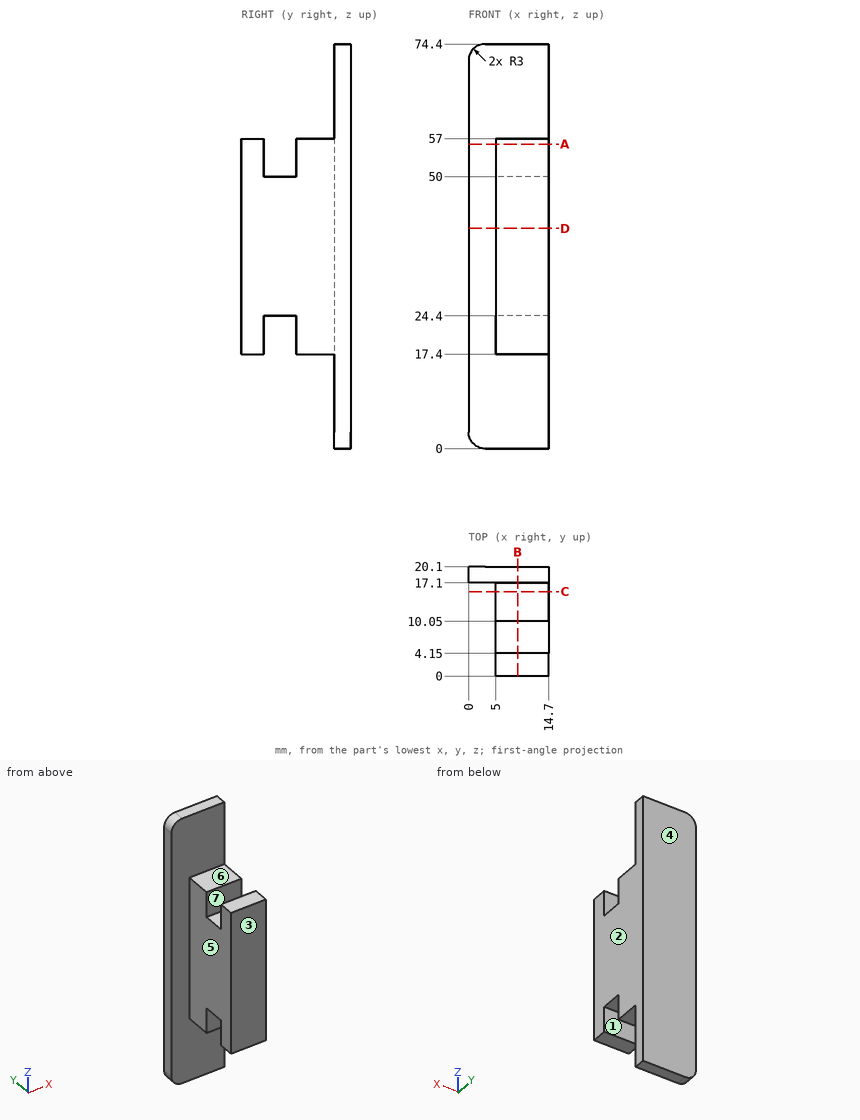
Check sheet for the drawn part. Datum: minimum x, y, z corner. Units: mm. A direction names the side the tool comes from. Coordinates: 2 decimals unless noted, no trailing zeros. Loops run counter-clockwise (first coordinate to the right, second up) from the corner with the lowest first, then second, coordinate; pieces in that order, holes last. Notation, with made-up numbers: (7, 12.25) -> (36, 12.25) arc R12 cw to (36, 23.25) -> close; hole circle Ø11 at (-38.5, 10). An arc over 180 degrees is marked (long way). Answer in a Markdown table with one row per item.
1. Sectioned sample at B-B, the plane x = 9. Record the boundary of the cut face in (y, z).
Check values:
| item | result |
|---|---|
| outline | (0, 17.4) -> (4.15, 17.4) -> (4.15, 24.4) -> (10.05, 24.4) -> (10.05, 17.4) -> (17.1, 17.4) -> (17.1, 0) -> (20.1, 0) -> (20.1, 74.4) -> (17.1, 74.4) -> (17.1, 57) -> (10.05, 57) -> (10.05, 50) -> (4.15, 50) -> (4.15, 57) -> (0, 57) -> close |
2. Go/stop test with flat-tipped pins: pin 1 (1 mm diameter, centred on x = 3, z = 15.5, fed in from -Y); pin 2 (5.5 mm diameter, centred on x = 8.5, y = 13.5, fed in from -Z); pin 3 (3 mm diameter, centred on x = 10, y = 6.5, fed in from +Z). Record where each tip stops, or that it passes through.
Check values:
| item | result |
|---|---|
| pin 1 | stops at y = 17.1 |
| pin 2 | stops at z = 17.4 |
| pin 3 | stops at z = 50 |
3. Material ranges on line 1 along Y through (x, z) = (8.25, 4); line 2 along X through (y, z) = (16, 27.5); line 3 along Z through (x, y) = (6, 12.5), recorded low to high. Write a range as [from, to].
Check values:
| item | result |
|---|---|
| line 1 | y = [17.1, 20.1] |
| line 2 | x = [5, 14.7] |
| line 3 | z = [17.4, 57] |
4. Sectioned sample at C-C, the plane y = 15.5. Record the boundary of the cut face in (x, z).
Check values:
| item | result |
|---|---|
| outline | (5, 17.4) -> (14.7, 17.4) -> (14.7, 57) -> (5, 57) -> close |
5. Release check for a two-part mould opening along Y. For the marked faces 1, 2 and 3 record: released by +Y, released by -Y, zero draft, split by the parting line, or undercut.
Check values:
| item | result |
|---|---|
| face 1 | undercut |
| face 2 | zero draft |
| face 3 | released by -Y |
6. Sectioned sample at A-A, the plane z = 56. Record the boundary of the cut face in (x, y).
Check values:
| item | result |
|---|---|
| outline | (0, 17.1) -> (5, 17.1) -> (5, 10.05) -> (14.7, 10.05) -> (14.7, 20.1) -> (0, 20.1) -> close; (5, 0) -> (14.7, 0) -> (14.7, 4.15) -> (5, 4.15) -> close |
7. Sectioned sample at D-D, the plane z = 40.5. Record the boundary of the cut face in (x, y).
Check values:
| item | result |
|---|---|
| outline | (0, 17.1) -> (5, 17.1) -> (5, 0) -> (14.7, 0) -> (14.7, 20.1) -> (0, 20.1) -> close |
8. Access from +Z, -Z, +X, -X, +Y, -Y to the whole of each face (thin tool, end or side, straight path). Record for the marked faces 4, 5, 6 and 7.
Check values:
| item | result |
|---|---|
| face 4 | +Z, -Z, +X, -X, +Y |
| face 5 | +Z, -Z, -X, -Y |
| face 6 | +Z, +X, -X, -Y |
| face 7 | +Z, +X, -X |
